```python
from build123d import *

# Parameters (mm, degrees)
EXTRUDE_1_DEPTH     = 35.6
SKETCH_3_R          = 1.5
SKETCH_3_W          = 20
SKETCH_3_H          = 35
CUT_EXTRUDE_1_DEPTH = 54.219921082
SKETCH_4_R          = 1.5
CUT_EXTRUDE_2_DEPTH = 54.219921082
FILLET_1_R          = 3
SKETCH_6_R          = 5.41
SKETCH_6_R_2        = 1.5
SKETCH_6_R_3        = 5.408326913
EXTRUDE_2_DEPTH     = 3
FILLET_2_R          = 3
SKETCH_7_W          = 3
SKETCH_7_H          = 15
CUT_EXTRUDE_3_DEPTH = 59


with BuildPart() as part:
    # Sketch 1 → Extrude 1 (new body)
    with BuildSketch(Plane.XY):
        Polygon((0, 0), (3, 0), (3, 35), (11, 35), (11, 38), (0, 38), align=None)
    extrude(amount=EXTRUDE_1_DEPTH)

    # Sketch 3 → Cut-Extrude 1 (cut, through all)
    with BuildSketch(Plane.ZY):
        with Locations((3.3, 3)):
            Circle(SKETCH_3_R)
        with Locations(Location((32.3, 3, 0), (0, 0, 270))):
            Circle(SKETCH_3_R)
        with Locations((17.8, 17.5)):
            Rectangle(SKETCH_3_W, SKETCH_3_H)
    extrude(amount=-CUT_EXTRUDE_1_DEPTH, mode=Mode.SUBTRACT)

    # Sketch 4 → Cut-Extrude 2 (cut, through all)
    with BuildSketch(Plane(origin=(0, 38, 0), x_dir=(1, 0, 0), z_dir=(0, 1, 0))):
        with Locations(Location((5.094069653, -7.8, 0), (0, 0, 270))):
            Circle(SKETCH_4_R)
        with Locations(Location((5.094069653, -27.8, 0), (0, 0, 270))):
            Circle(SKETCH_4_R)
    extrude(amount=-CUT_EXTRUDE_2_DEPTH, mode=Mode.SUBTRACT)

    # Fillet 1
    fillet_1_edges = [part.edges().sort_by_distance(p)[0] for p in [
        (11, 36.5, 35.6),
        (11, 36.5, 0),
    ]]
    fillet(fillet_1_edges, radius=FILLET_1_R)

    # Sketch 6 → Extrude 2 (add)
    # profile 1 of 2: a face of its own
    with BuildSketch(Plane.ZY):
        with Locations((3.3, 3)):
            Circle(SKETCH_6_R)
        with Locations((3.3, 3)):
            Circle(SKETCH_6_R_2, mode=Mode.SUBTRACT)
    # profile 2 of 2: a face of its own
    with BuildSketch(Plane.ZY):
        with Locations((32.3, 3)):
            Circle(SKETCH_6_R_3)
        with Locations(Location((32.3, 3, 0), (0, 0, 270))):
            Circle(SKETCH_6_R_2, mode=Mode.SUBTRACT)
    extrude(amount=-EXTRUDE_2_DEPTH)

    # Fillet 2
    fillet_2_edges = [part.edges().sort_by_distance(p)[0] for p in [
        (1.5, 6.003015151, 7.8),
        (1.5, 7.286968626, 0),
        (1.5, 6, 27.8),
        (1.5, 7.284857057, 35.6),
    ]]
    fillet(fillet_2_edges, radius=FILLET_2_R)

    # Sketch 7 → Cut-Extrude 3 (cut)
    with BuildSketch(Plane.XY.offset(35.6)):
        with Locations((1.5, 25.41705132)):
            Rectangle(SKETCH_7_W, SKETCH_7_H)
    extrude(amount=-CUT_EXTRUDE_3_DEPTH, mode=Mode.SUBTRACT)


with BuildPart() as cut_extrude_3_piece_1:
    # of the separate pieces the step leaves, piece 1, a body of its own (cut_extrude_3_pieces)
    add(part.part.solids().sort_by_distance((0, 32.91705132, 0))[0])


with BuildPart() as cut_extrude_3_piece_2:
    # of the separate pieces the step leaves, piece 2, a body of its own (cut_extrude_3_pieces)
    add(part.part.solids().sort_by_distance((3, 8.571184793, 0))[0])


with BuildPart() as cut_extrude_3_piece_3:
    # of the separate pieces the step leaves, piece 3, a body of its own (cut_extrude_3_pieces)
    add(part.part.solids().sort_by_distance((0, 17.91705132, 35.6))[0])


with BuildPart() as cut_extrude_3_piece_1_1:
    # Move Body 1: moved
    add(cut_extrude_3_piece_1.part.moved(Location((0, -15, 0))))

    # Combine 3: union Cut-Extrude 3 piece 2, Cut-Extrude 3 piece 3
    add(cut_extrude_3_piece_2.part)
    add(cut_extrude_3_piece_3.part)


solid = cut_extrude_3_piece_1_1.part
```
Check sheet for the modelled part. Datum: model origin and axes. Units: mm. A direction names the side the tool comes from. Coordinates: 2 decimals unless noted, no trailing zeros. Order: outer loops, then holes, each group sorted by start corner. A loop starts at its lowest first (then second) coordinate and runs counter-clockwise, first axis right, second up. Notation, with made-up numbers: (88.25, 40) -> (110.25, 40) arc R35 cw to (110.25, 72) -> close; hole circle Ø10 at (6, 1). An arc over 180 degrees is marked (long way). Write each question's results on one line, items separated by ' | '. Start each with the question number.
1) Set-up check for faces 1 (the face through (1, 13, 27.8)), 2 (the face through (1.48, 7.49, 35.8)), 3 (the face through (2, 17, 0)), 4 (the face through (3, 9, 3)): record each of +Z, -Z, +X, -X, +Y, -Y from which the full face is reachable in a straight line by a thin tool's end or side.
2) Section check A-A (y = 17.5). Enter the section's corners in (x, z), and give its area (3 significant figures).
3) Section check D-D (z = 28.5). Enter the section's corners in (x, y), and give its area (3 significant figures).
4) Material ranges on line 1 along Y through (x, z) = (2.3, 3.3); line 2 along Y through (x, z) = (9, 19.5); line 3 along Z through (x, y) = (2, 8.5), recorded low to high.
5) Section check B-B (x = 2). Enter the section's corners in (y, z) (3 decimals).
6) Draft check along Z on faces 5 (the face through (4.18, 21.52, 6.61)), 6 (the face through (3, 9, 32)), 7 (the face through (1.48, 7.49, -0.2)), 8 (the face through (1, 13, 7.8)). Enter one of: pulls with the +Z half, pulls with the -Z half, needs draft (parallel to the pull), parting line crosses it, or undercut.
7) Section check C-C (y = 3). Enter the section's corners in (x, z).
8) Depth check by flat-ended pin: pin 1 (6 mm diameter, centred on y = 15.5, z = 15.5, fed in from +X); pin 2 (5.5 mm diameter, centred on y = 8.5, z = 3, fed in from +X); pin 3 (1.5 mm diameter, centred on x = 2, y = 13, fed in from +Z); pin 4 (3.5 mm diameter, centred on x = 7, z = 19, fed in from -Y). Enter the tip coordinate at first touch or a pass-through.
Checked values:
1) face 1: +X, -X | face 2: +Z, +X, -X, +Y | face 3: -Z, +X, -X, +Y | face 4: +Z, -Z, +X, -Y
2) outline: (0, 0) -> (3, 0) -> (3, 7.8) -> (0, 7.8) -> close; (0, 27.8) -> (3, 27.8) -> (3, 35.6) -> (0, 35.6) -> close | area: 46.8 mm²
3) outline: (0, -0.85) -> (3, -0.85) -> (3, 20) -> (3.77, 20) -> (3.77, 23) -> (0, 23) -> close; (6.42, 20) -> (11, 20) -> (11, 23) -> (6.42, 23) -> close | area: 87.6 mm²
4) line 1: -2.41 to 1.5, 4.5 to 23 | line 2: 20 to 23 | line 3: 0 to 7.8, 27.8 to 35.6
5) outline: (5.445, 27.476) arc R3 cw to (6.801, 27.8) -> (20, 27.8) -> (20, 7.8) -> (6.805, 7.8) arc R3 cw to (5.448, 8.125) arc R5.41 ccw (long way) to (6.584, -0.753) arc R3 cw to (8.571, 0) -> (23, 0) -> (23, 35.6) -> (8.569, 35.6) arc R3 cw to (6.582, 36.352) arc R5.408 ccw (long way) to start; hole circle Ø3 at (3, 3.3); hole circle Ø3 at (3, 32.3)
6) face 5: undercut | face 6: needs draft | face 7: pulls with the -Z half | face 8: undercut
7) outline: (0, -2.11) -> (3, -2.11) -> (3, 1.8) -> (0, 1.8) -> close; (0, 4.8) -> (3, 4.8) -> (3, 8.71) -> (0, 8.71) -> close; (0, 26.89) -> (3, 26.89) -> (3, 30.8) -> (0, 30.8) -> close; (0, 33.8) -> (3, 33.8) -> (3, 37.71) -> (0, 37.71) -> close
8) pin 1: through | pin 2: x = 3 | pin 3: z = 35.6 | pin 4: y = 20
